Build history of the part. All positions in model axes, mm. A direction names the side the tool comes from. Coordinates: 2 decimals unless noted, no trailing zeros. One line per item, written item: value.
from build123d import *

# Parameters (mm, degrees)
SKETCH1_W           = 600
SKETCH1_H           = 610
BOSS_EXTRUDE1_DEPTH = 600
SKETCH2_W           = 560
SKETCH2_H           = 140
SKETCH2_W_2         = 80
SKETCH2_H_2         = 20
SKETCH2_H_3         = 436.439883301
SKETCH2_W_3         = 20
SKETCH2_H_4         = 80
BOSS_EXTRUDE2_DEPTH = 10


with BuildPart() as part:
    # Sketch1 → Boss-Extrude1 (new body)
    with BuildSketch(Plane.XY):
        with Locations((-300, -305)):
            Rectangle(SKETCH1_W, SKETCH1_H)
    extrude(amount=BOSS_EXTRUDE1_DEPTH)

    # Sketch2 → Boss-Extrude2 (add)
    with BuildSketch(Plane(origin=(0, 0, 0), x_dir=(0, 0, -1), z_dir=(1, 0, 0))):
        with Locations((-300, -79.996604702)):
            Rectangle(SKETCH2_W, SKETCH2_H)
        with Locations((-292, -79.960529666)):
            Rectangle(SKETCH2_W_2, SKETCH2_H_2, mode=Mode.SUBTRACT)
        with Locations((-300, -383.216546353)):
            Rectangle(SKETCH2_W, SKETCH2_H_3)
        with Locations((-560, -383.759018759)):
            Rectangle(SKETCH2_W_3, SKETCH2_H_4, mode=Mode.SUBTRACT)
    extrude(amount=BOSS_EXTRUDE2_DEPTH)


solid = part.part
1. Flat gauge pins, fed straight in: P1, Ø3, axis at x = 3.5, y = -343, coming from the +Z side; P2, Ø5, axis at x = 4.5, z = 379.5, coming from the +Y side; P3, Ø3, axis at x = 6.5, y = -79.5, coming from the -Z side. Where does each tip first touch, or does it go through?
Values found:
P1: stops at z = 580
P2: stops at y = -10
P3: stops at z = 20
2. Two-plate mould, pull along Y, no slides. Class faces 3 (the face through (-304, 0, 296)), 4 (the face through (0, -80, 291)), 5 (the face through (10, -63, 304)): pulls with the +Y half, pulls with the -Y half, needs draft (parallel to the pull), parting line crosses it, or undercut.
Values found:
face 3: pulls with the +Y half
face 4: undercut
face 5: needs draft
3. 3-axis set-ups, long thin cutter, end or side, ignore diameter. For faces 1 (the face through (0, -384, 560)), 2 (the face through (-304, -301, 600)): which of +Z, -Z, +X, -X, +Y, -Y reach the whole face in a straight line?
Values found:
face 1: +X
face 2: +Z, +X, -X, +Y, -Y
4. Probe line 1 along X through (y, z) = (-161.5, 255.5). List the from-to ranges inside material, lowest first.
Values found:
line 1: x = -600 to 0
